Part model, mm, in its own coordinate system. Face numbers are marked on the shaded views. A direction names the side the tool comes from. Give positions to 0.01 mm unless a question says otherwise; leave off trailing zeros. Write each loop counter-clockwise with the first axis right and the second up, starting at its lowest first coordinate (ties: lowest second). Pieces come first, ordered by that corner, then holes. Notation, with made-up numbers: (-2, -3.5) - (3, -3.5) arc R15 cw to (3, 6.5) - close; hole circle Ø2 at (36, 70.25). An arc over 180 degrees is marked (long way). Answer in a Markdown table with one row per item. Add a question column.
1. Probe line 1 along Z through (x, y) = (14, 4.5); line 2 along Y through (x, z) = (-1, 10.25); line 3 along X through (y, z) = (-1, 11). List the from-to ranges inside material, lowest first.
2. Band-saw the part on A-A on x = 0. Write the cut outline in (y, z), plus the area to 3 significant figures.
3. Which spindle directions (+Z, -Z, +X, -X, +Y, -Y) get a long thin tool onto all of the face, cutting with end or side? Do the marked faces 1, 2 and 3. Say none if no direction does.
4. Band-saw the part on B-B on z = 14.25. Write the cut outline in (x, y), plus the area to 3 significant figures.
5. Drop flat-ended pins along their axis: pin 1 Ø3 at (y, z) = (0.5, 3) entering from +X; pin 2 Ø12 at (y, z) = (12.5, 12.5) entering from +X; pin 3 Ø1 at (x, y) = (-9, -3.5) entering from +Z; pin 4 Ø1 at (x, z) = (-7.5, 7) entering from -Y. Give the stop position or say it passes through.
```python
from build123d import *

# Parameters (mm, degrees)
F0_R     = 18.75
F1_DEPTH = 5
F2_R     = 7.75
F3_DEPTH = 20
F4_SIZE  = 0.5
F5_SIZE  = 1


with BuildPart() as f1:
    # F0 (on Top) → F1 (new body)
    with BuildSketch(Plane.XY):
        Circle(F0_R)
        Polygon((2.598076, 4.5), (5.196152, 0), (2.598076, -4.5), (-2.598076, -4.5), (-5.196152, 0), (-2.598076, 4.5), align=None, mode=Mode.SUBTRACT)
    extrude(amount=F1_DEPTH)

    # F2 (on face) → F3 (join)
    with BuildSketch(Plane.XY.offset(5)):
        Circle(F2_R)
        Polygon((-2.598076, -4.5), (-5.196152, 0), (-2.598076, 4.5), (2.598076, 4.5), (5.196152, 0), (2.598076, -4.5), align=None, mode=Mode.SUBTRACT)
    extrude(amount=F3_DEPTH)

    # F4
    f4_edges = [f1.edges().sort_by_distance(p)[0] for p in [
        (-18.75, 0, 0),
        (-18.75, 0, 5),
    ]]
    chamfer(f4_edges, length=F4_SIZE)

    # F5
    f5_edges = [f1.edges().sort_by_distance(p)[0] for p in [
        (-7.75, 0, 25),
    ]]
    chamfer(f5_edges, length=F5_SIZE)


solid = f1.part
```
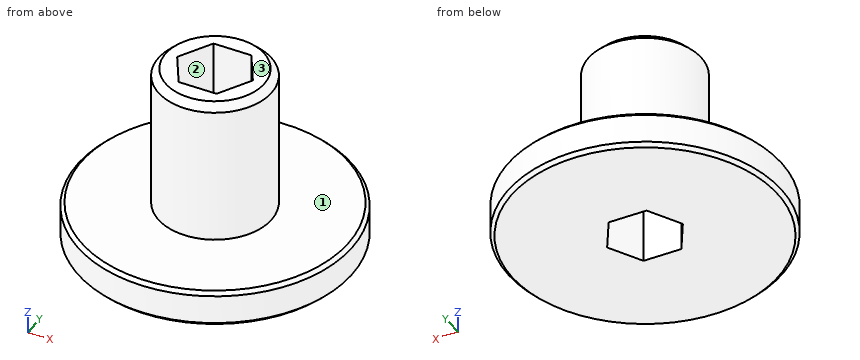
Values:
| question | item | result |
|---|---|---|
| 1 | line 1 | z = 0 to 5 |
| 1 | line 2 | y = -7.69 to -4.5, 4.5 to 7.69 |
| 1 | line 3 | x = -7.69 to -4.62, 4.62 to 7.69 |
| 2 | outline | (-18.75, 0.5) - (-18.25, 0) - (-4.5, 0) - (-4.5, 25) - (-6.75, 25) - (-7.75, 24) - (-7.75, 5) - (-18.25, 5) - (-18.75, 4.5) - close; (4.5, 0) - (18.25, 0) - (18.75, 0.5) - (18.75, 4.5) - (18.25, 5) - (7.75, 5) - (7.75, 24) - (6.75, 25) - (4.5, 25) - close |
| 2 | area | 271 mm² |
| 3 | face 1 | +Z |
| 3 | face 2 | +Z, -Z |
| 3 | face 3 | +Z, +X, -X, +Y, -Y |
| 4 | outline | circle Ø15.5 at (0, 0); hole (-5.2, 0) - (-2.6, -4.5) - (2.6, -4.5) - (5.2, 0) - (2.6, 4.5) - (-2.6, 4.5) - close |
| 4 | area | 119 mm² |
| 5 | pin 1 | stops at x = 18.75 |
| 5 | pin 2 | stops at x = 4.22 |
| 5 | pin 3 | stops at z = 5 |
| 5 | pin 4 | stops at y = -3.33 |
